Model file for the job. Use its own axes, mm. A direction names the side the tool comes from. Coordinates: 2 decimals unless noted, no trailing zeros. Write each loop counter-clockwise with the first axis right and the second up, starting at its lowest first coordinate (ties: lowest second). Pieces come first, ordered by that corner, then holes.
Q1. Band-saw the part on D-D, the plane x = 2.5. Write the cut outline in (y, z), plus the area to 3 significant figures.
Q2. Band-saw the part on A-A, the plane y = -20.2. Write the cut outline in (x, z), plus the area to 3 significant figures.
Q3. Band-saw the part on C-C, the plane y = -2.5. Write the cut outline in (x, z).
Q4. Which spindle directions (+Z, -Z, +X, -X, +Y, -Y) get a long thin tool onto all of the face, cutting with end or side? Do faces 5 (the cylindrical face through (-1, -17, 8)), 6 (the flat face through (-1, -17, 12)), 7 (the flat face through (-1, 6, 26)), 8 (the flat face through (4, -16, 10.9)). Say none if no direction does.
Q5. Pin check, flat tips, straight feed: P1, Ø5, axis at x = -1, z = 30.5, coming from the +Y side; P2, Ø6, axis at x = -2, y = -11.5, coming from the -Z side; P3, Ø1.9, axis at x = -1, y = -11, coming from the -Z side; P4, Ø2.5, axis at x = -2, y = 8.5, coming from the +Z side. Stop position of each tip, or through.
Q6. Drill centre lines: probe 1 along Y at (x, z) = (-1, 2.55) (3 decimals); probe 2 along X at (y, z) = (9.2, 15.2); probe 3 along Z at (x, y) = (-1.25, -11.5). Where is each one in solid material? Low to high.
Q7. Band-saw the part on B-B, the plane z = 14. Write the cut outline in (x, y), plus the area to 3 significant figures.
Q8. Pull direction X, two halves, no side cores. Call faces 1 (the cylindrical face through (-1.713, -8.735, 3.374)), 2 (the cylindrical face through (-0.95, -18.95, 14.98)), 3 (the flat face through (2, 11, 15)), 4 (the cylindrical face through (-1.05, 7.95, 14.98)): released by +X, released by -X, zero draft, split by the parting line, or undercut.
from build123d import *

# Parameters (mm, degrees)
SKETCH063_W             = 23
SKETCH063_H             = 12
PAD032_DEPTH            = 23.5
SKETCH064_W             = 5
SKETCH064_H             = 12
PAD033_DEPTH            = 2.8
POCKET026_DEPTH         = 5
PAD034_DEPTH            = 5.8
SKETCH067_R             = 2.375
SKETCH067_R_2           = 1.2
PAD035_DEPTH            = 3.5
BODY010_ROLL_ANGLE      = -90
BODY010_PLACEMENT_ANGLE = 90


with BuildPart() as part:
    # Sketch063 → Pad032 (new body)
    with BuildSketch(Plane.XZ):
        with Locations((11.5, 6)):
            Rectangle(SKETCH063_W, SKETCH063_H)
    extrude(amount=-PAD032_DEPTH)

    # Sketch064 → Pad033 (join)
    with BuildSketch(Plane.XZ.offset(-18)):
        with Locations((-2.5, 6)):
            Rectangle(SKETCH064_W, SKETCH064_H)
        with Locations((25.5, 6)):
            Rectangle(SKETCH064_W, SKETCH064_H)
    extrude(amount=-PAD033_DEPTH)

    # Sketch065 → Pocket026 (cut)
    with BuildSketch(Plane(origin=(-3.2, 20.8, 6), x_dir=(1, 0, 0), z_dir=(0, -1, 0))):
        with BuildLine():
            ThreePointArc((-1.096586, -0.6), (1.25, 0), (-1.096586, 0.6))
            Line((-1.8, 0.6), (-1.096586, 0.6))
            Line((-1.8, 0), (-1.8, 0.6))
            Line((-1.8, 0), (-1.8, -0.6))
            Line((-1.8, -0.6), (-1.096586, -0.6))
        make_face()
        with BuildLine():
            ThreePointArc((30.496586, 0.6), (28.15, 0), (30.496586, -0.6))
            Line((31.2, -0.6), (30.496586, -0.6))
            Line((31.2, 0), (31.2, -0.6))
            Line((31.2, 0), (31.2, 0.6))
            Line((31.2, 0.6), (30.496586, 0.6))
        make_face()
    extrude(amount=POCKET026_DEPTH, mode=Mode.SUBTRACT)

    # Sketch066 → Pad034 (join)
    with BuildSketch(Plane(origin=(6, 23.5, 6), x_dir=(1, 0, 0), z_dir=(0, -1, 0))):
        with BuildLine():
            ThreePointArc((5.25, 2.904738), (-6, 0), (5.25, -2.904738))
            ThreePointArc((5.25, -2.904738), (9, 0), (5.25, 2.904738))
        make_face()
    extrude(amount=-PAD034_DEPTH)

    # Sketch067 → Pad035 (join)
    with BuildSketch(Plane(origin=(6, 29.3, 6), x_dir=(1, 0, 0), z_dir=(0, -1, 0))):
        Circle(SKETCH067_R)
        Circle(SKETCH067_R_2, mode=Mode.SUBTRACT)
    extrude(amount=-PAD035_DEPTH)


with BuildPart() as part_1:
    # Body010 roll: moved
    add(part.part.rotate(Axis((0, 0, 0), (1, 0, 0)), BODY010_ROLL_ANGLE))


with BuildPart() as part_2:
    # Body010 placement: moved
    add(part_1.part.moved(Location((5, -17, 34.4))).rotate(Axis((5, -17, 34.4), (0, 0, 1)), BODY010_PLACEMENT_ANGLE))


solid = part_2.part
Answer sheet:
1. outline: (-22, 13.6) - (-17, 13.6) - (-17, 10.9) - (-15.87, 10.9) - (-15.87, 5.1) - (-6.13, 5.1) - (-6.13, 10.9) - (6, 10.9) - (6, 13.6) - (11, 13.6) - (11, 16.4) - (6, 16.4) - (6, 34.4) - (-17, 34.4) - (-17, 16.4) - (-22, 16.4) - close
1. area: 625 mm2
2. outline: (-7, 13.6) - (-2.25, 13.6) - (-2.25, 16.4) - (-7, 16.4) - close; (0.25, 13.6) - (5, 13.6) - (5, 16.4) - (0.25, 16.4) - close
2. area: 26.6 mm2
3. outline: (-7, 10.9) - (-2.66, 10.9) - (-2.66, 5.1) - (0.66, 5.1) - (0.66, 10.9) - (5, 10.9) - (5, 34.4) - (-7, 34.4) - close
4. face 5: -Z
4. face 6: -Z, +X, -X, -Y
4. face 7: +Z, +X, -X, +Y
4. face 8: -Z, +X, -Y
5. P1: stops at y = 6
5. P2: stops at z = 1.6
5. P3: stops at z = 5.1
5. P4: stops at z = 16.4
6. probe 1: y = -13.375 to -12.2, -9.8 to -8.625
6. probe 2: x = -7 to -2.25, 0.25 to 5
6. probe 3: z = 5.1 to 34.4
7. outline: (-7, -22) - (-1.6, -22) - (-1.6, -21.3) arc R1.25 cw (long way) to (-0.4, -21.3) - (-0.4, -22) - (5, -22) - (5, 11) - (-0.4, 11) - (-0.4, 10.3) arc R1.25 cw (long way) to (-1.6, 10.3) - (-1.6, 11) - (-7, 11) - close
7. area: 385 mm2
8. face 1: split by the parting line
8. face 2: undercut
8. face 3: zero draft
8. face 4: undercut
